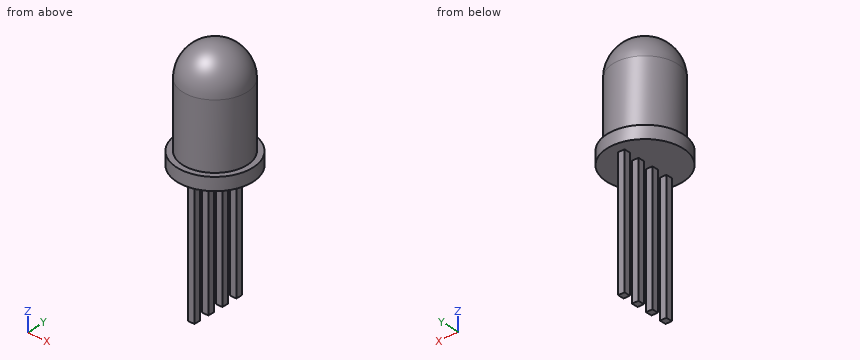
Autodesk Inventor part; units mm, degrees
ref_plane "YZ Plane" through (0, 0, 0) normal (1, 0, 0) x (0, 1, 0)
ref_plane "XZ Plane" through (0, 0, 0) normal (0, 1, 0) x (-1, 0, 0)
ref_plane "XY Plane" through (0, 0, 0) normal (0, 0, 1) x (1, 0, 0)
sketch "스케치1" plane through (0, 0, 0) normal (1, 0, 0) x (0, 1, 0)
  line L0 (0, 0) -> (0, -8.6)
  line L1 (0, -8.6) -> (0, -25.7335)
  arc A0 (2.5, -2.5) -> (0, 0) centre (0, -2.5) ccw
  line L2 (2.5, -2.5) -> (2.5, -7.6)
  line L3 (0, -8.6) -> (2.95, -8.6)
  line L4 (2.95, -8.6) -> (2.95, -7.6)
  line L5 (2.95, -7.6) -> (2.5, -7.6)
  dimension "d0" = 8.6
  dimension "d1" = 17.1335
  dimension "d2" = 5
  dimension "d3" = 1
  dimension "d4" = 2.5
  dimension "d6" = 5.9
revolve "회전1" add sketch "스케치1" angle 360 about axis through (0, 0, -8.6) along (0, 0, -1)
sketch "스케치2" plane through (0, 0, -8.6) normal (0, 0, -1) x (-1, 0, 0)
  line L0 (0.25, -1.655) -> (-0.25, -1.655)
  line L1 (-0.25, -1.655) -> (-0.25, -2.155)
  line L2 (-0.25, -2.155) -> (0.25, -2.155)
  line L3 (0.25, -2.155) -> (0.25, -1.655)
  line L4 (0.25, -1.655) -> (-0.25, -2.155) construction
  line L5 (-0.25, -1.655) -> (0.25, -2.155) construction
  line L6 (0.25, -0.385) -> (-0.25, -0.385)
  line L7 (-0.25, -0.385) -> (-0.25, -0.885)
  line L8 (-0.25, -0.885) -> (0.25, -0.885)
  line L9 (0.25, -0.885) -> (0.25, -0.385)
  line L10 (0.25, -0.385) -> (-0.25, -0.885) construction
  line L11 (-0.25, -0.385) -> (0.25, -0.885) construction
  line L12 (0.25, 0.885) -> (-0.25, 0.885)
  line L13 (-0.25, 0.885) -> (-0.25, 0.385)
  line L14 (-0.25, 0.385) -> (0.25, 0.385)
  line L15 (0.25, 0.385) -> (0.25, 0.885)
  line L16 (0.25, 0.885) -> (-0.25, 0.385) construction
  line L17 (-0.25, 0.885) -> (0.25, 0.385) construction
  line L18 (0.25, 2.155) -> (-0.25, 2.155)
  line L19 (-0.25, 2.155) -> (-0.25, 1.655)
  line L20 (-0.25, 1.655) -> (0.25, 1.655)
  line L21 (0.25, 1.655) -> (0.25, 2.155)
  line L22 (0.25, 2.155) -> (-0.25, 1.655) construction
  line L23 (-0.25, 2.155) -> (0.25, 1.655) construction
  line L24 (0, -1.905) -> (0, 1.905) construction
  point P0 (0, 0)
  point P1 (0, -0.635)
  point P2 (0, 0.635)
  point P3 (0, 0)
  point P4 (0, 0)
  dimension "d8" = 0.5
  dimension "d9" = 0.5
  dimension "d10" = 0.5
  dimension "d11" = 0.5
  dimension "d12" = 0.5
  dimension "d13" = 0.5
  dimension "d14" = 0.5
  dimension "d15" = 0.5
  dimension "d16" = 1.27
  dimension "d17" = 1.27
  dimension "d18" = 1.27
extrude "돌출1" add sketch "스케치2" along normal blind 10
properties part number "led"
Geometry check sheet. Reference: the model listing, model coordinates, mm. Coordinates: 2 decimals unless noted, no trailing zeros. Order: outer loops, then holes, each group sorted by start corner. A loop starts at its lowest first (then second) coordinate and runs counter-clockwise, first axis right, second up. Notation, with made-up numbers: (13.5, 35) -> (72.5, 35) arc R22 cw to (72.5, 70) -> close; hole circle Ø8 at (-32.75, 11). An arc over 180 degrees is marked (long way). Use a Markdown table: item, result. Add a question column.
1. Cross-section at C-C (x = 0). Enter the section's corners in (y, z) (3 decimals).
2. Cross-section at A-A (z = -9.5). Enter the section's corners in (x, y) (3 decimals).
3. Go/stop test with flat-tipped pins: pin 1 Ø0.5 at (y, z) = (2, -13) entering from +X; pin 2 Ø0.6 at (y, z) = (0.5, -15.5) entering from -X; pin 3 Ø0.6 at (x, z) = (0, -14) entering from +Y (3 decimals). Record where each tip stops, or that it passes through.
4. Cross-section at D-D (x = -1.95). Enter the section's corners in (y, z), and give its area (3 significant figures).
5. Cross-section at B-B (y = 0). Enter the section's corners in (x, z).
6. Material ranges on L1, parallel to Y at x = -0.1, z = -13.25 (3 decimals); L2, parallel to X at y = -0.8, z = -12.25; L3, parallel to Z at x = 0.2, y = 2.65, recorded low to high.
Filled sheet:
| question | item | result |
|---|---|---|
| 1 | outline | (-2.95, -8.6) -> (-2.155, -8.6) -> (-2.155, -18.6) -> (-1.655, -18.6) -> (-1.655, -8.6) -> (-0.885, -8.6) -> (-0.885, -18.6) -> (-0.385, -18.6) -> (-0.385, -8.6) -> (0.385, -8.6) -> (0.385, -18.6) -> (0.885, -18.6) -> (0.885, -8.6) -> (1.655, -8.6) -> (1.655, -18.6) -> (2.155, -18.6) -> (2.155, -8.6) -> (2.95, -8.6) -> (2.95, -7.6) -> (2.5, -7.6) -> (2.5, -2.5) arc R2.5 ccw to (-2.5, -2.5) -> (-2.5, -7.6) -> (-2.95, -7.6) -> close |
| 2 | outline | (-0.25, -2.155) -> (0.25, -2.155) -> (0.25, -1.655) -> (-0.25, -1.655) -> close; (-0.25, -0.885) -> (0.25, -0.885) -> (0.25, -0.385) -> (-0.25, -0.385) -> close; (-0.25, 0.385) -> (0.25, 0.385) -> (0.25, 0.885) -> (-0.25, 0.885) -> close; (-0.25, 1.655) -> (0.25, 1.655) -> (0.25, 2.155) -> (-0.25, 2.155) -> close |
| 3 | pin 1 | x = 0.25 |
| 3 | pin 2 | x = -0.25 |
| 3 | pin 3 | y = 2.155 |
| 4 | outline | (-2.21, -8.6) -> (2.21, -8.6) -> (2.21, -7.6) -> (1.56, -7.6) -> (1.56, -2.5) arc R1.56 ccw to (-1.56, -2.5) -> (-1.56, -7.6) -> (-2.21, -7.6) -> close |
| 4 | area | 24.2 mm2 |
| 5 | outline | (-2.95, -8.6) -> (2.95, -8.6) -> (2.95, -7.6) -> (2.5, -7.6) -> (2.5, -2.5) arc R2.5 ccw to (-2.5, -2.5) -> (-2.5, -7.6) -> (-2.95, -7.6) -> close |
| 6 | L1 | -2.155 to -1.655, -0.885 to -0.385, 0.385 to 0.885, 1.655 to 2.155 |
| 6 | L2 | -0.25 to 0.25 |
| 6 | L3 | -8.6 to -7.6 |
